from build123d import *

# Parameters (mm, degrees)
BASE_FLANGE1_DEPTH = 2
FILLET1_R          = 10


# Sheet-metal steps are written as plain solids
with BuildPart() as part:
    # Sketch1 → Base-Flange1 (new body)
    with BuildSketch(Plane.XY):
        Polygon((-65, 15), (-75, 15), (-75, 79), (29, 79), (29, -75), (-65, -75), align=None)
    extrude(amount=-BASE_FLANGE1_DEPTH)

    # Fillet1
    fillet1_edges = [part.edges().sort_by_distance(p)[0] for p in [
        (-75, 79, -1),
        (-75, 15, -1),
        (-65, -75, -1),
        (29, -75, -1),
        (29, 79, -1),
    ]]
    fillet(fillet1_edges, radius=FILLET1_R - 0.0001)  # a hair under: the kernel refuses the full size


solid = part.part
Could you check a few things on this model? Use its own coordinates, in mm. Round coordinates to 2 decimals unless told otherwise and drop trailing zeros. Order: outer loops, then holes, each group sorted by start corner. A loop starts at its lowest first (then second) coordinate and runs counter-clockwise, first axis right, second up.
Q1. Imagine slicing it at C-C, the plane x = -63. List the corners of the cut face in (y, z) for me, then the cut area to 3 significant figures.
Geometry says:
outline: (-71, -2) - (79, -2) - (79, 0) - (-71, 0) - close
area: 300 mm2
Q2. Please list where these lines run through material, in increasing order: probe 1 along X at (y, z) = (-29.5, -1.3); probe 2 along Y at (x, z) = (-60, -0.5); probe 3 along Y at (x, z) = (24.5, -1.9).
Geometry says:
probe 1: x = -65 to 29
probe 2: y = -73.66 to 79
probe 3: y = -73.35 to 77.35
Q3. I'm going to push a flat-ended pin straight in: P1, Ø10, axis at x = 18, y = -3.5, coming from the +Z side. Where does the tip first touch, or does it pass through?
Geometry says:
P1: stops at z = 0
Q4. Imagine slicing it at B-B, the plane y = 10. List the corners of the cut face in (x, z) for me.
Geometry says:
outline: (-65, -2) - (29, -2) - (29, 0) - (-65, 0) - close
